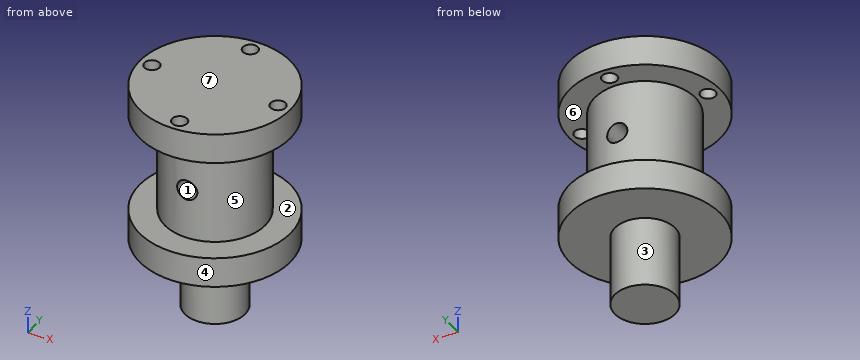
from build123d import *

# Parameters (mm, degrees)
BOSS_EXTRUDE1_DEPTH      = 5
BOSS_EXTRUDE1_DEPTH_BACK = 5
SKETCH1_R                = 5
SKETCH3_R                = 7.5
BOSS_EXTRUDE2_DEPTH      = 3
SKETCH4_R                = 1
CUT_EXTRUDE1_DEPTH       = 17.628289148
SKETCH5_R                = 0.75
CUT_EXTRUDE2_DEPTH       = 17.777961736
CIRPATTERN1_COUNT        = 4
SKETCH6_R                = 3
BOSS_EXTRUDE3_DEPTH      = 7


with BuildPart() as part:
    # Sketch1 → Boss-Extrude1 (new, two sides: drawn at the far end of the back side and taken through both)
    with BuildSketch(Plane.XY.offset(-BOSS_EXTRUDE1_DEPTH_BACK)):
        Circle(SKETCH1_R)
    extrude(amount=BOSS_EXTRUDE1_DEPTH + BOSS_EXTRUDE1_DEPTH_BACK)

    # Sketch3 → Boss-Extrude2 (add)
    with BuildSketch(Plane.XY.offset(5)):
        Circle(SKETCH3_R)
    boss_extrude2 = extrude(amount=BOSS_EXTRUDE2_DEPTH)

    # Mirror1: Boss-Extrude2 across plane
    add(boss_extrude2.mirror(Plane.XY))

    # Sketch4 → Cut-Extrude1 (cut, through all)
    with BuildSketch(Plane(origin=(0, 5, 0), x_dir=(1, 0, 0), z_dir=(0, 1, 0))):
        with Locations(Location((0, 0, 0), (0, 0, 270))):
            Circle(SKETCH4_R)
    extrude(amount=-CUT_EXTRUDE1_DEPTH, mode=Mode.SUBTRACT)

    # Sketch5 → Cut-Extrude2 (cut, through all)
    with BuildSketch(Plane(origin=(0, 0, 5), x_dir=(-1, 0, 0), z_dir=(0, 0, -1))):
        with Locations((0, 6.25)):
            Circle(SKETCH5_R)
    cut_extrude2 = extrude(amount=-CUT_EXTRUDE2_DEPTH, mode=Mode.SUBTRACT)

    # CirPattern1: Cut-Extrude2 ×4 about axis
    cirpattern1_axis = Axis((0, 0, 0), (0, 0, 1))
    for i in range(1, CIRPATTERN1_COUNT):
        add(cut_extrude2.rotate(cirpattern1_axis, i * 360 / CIRPATTERN1_COUNT), mode=Mode.SUBTRACT)

    # Sketch6 → Boss-Extrude3 (add)
    with BuildSketch(Plane(origin=(0, 0, -8), x_dir=(-1, 0, 0), z_dir=(0, 0, -1))):
        Circle(SKETCH6_R)
    extrude(amount=BOSS_EXTRUDE3_DEPTH)


solid = part.part
Verification items for the finished model (mm, model axes). Face numbers are marked on the shaded views. A direction names the side the tool comes from. Give positions to 0.01 mm unless a question says otherwise; leave off trailing zeros. Write each loop counter-clockwise with the first axis right and the second up, starting at its lowest first coordinate (ties: lowest second). Pieces come first, ordered by that corner, then holes. Notation, with made-up numbers: M -7,-30 L 1,-30 A7 ccw 1,-25 Z; hole C 44,17 d7. An arc over 180 degrees is marked long. Put each result on its own line as item: value. Start each with the question number.
1. Scan lines: line 1 along Z through (x, y) = (-2.25, 5.25); line 2 along X through (y, z) = (0.5, 7.25); line 3 along Z through (x, y) = (-3, -1.75). Record each from-to range of solid material in increasing order. Write a range as [from, to].
2. Draft check along Z on the marked faces 4, 5, 6 and 7. Enter one of: +Z half, -Z half, draft (parallel to the pull), parting line (faces both ways), or undercut.
3. Section check B-B (y = -2). Record the cut outline in (x, z), and give its area (3 significant figures).
4. Set-up check for the marked faces 1, 2 and 3: record each of +Z, -Z, +X, -X, +Y, -Y from which the full face is reachable in a straight line by a thin tool's end or side.
5. Section check C-C (y = -6.25). Record the cut outline in (x, z), and give its area (3 significant figures).
6. Section check A-A (y = 0). Record the cut outline in (x, z).
7. Go/stop test with flat-tipped pins: pin 1 Ø3 at (x, z) = (2.5, -10.5) entering from +Y; pin 2 Ø1.4 at (x, y) = (6.25, 0) entering from +Z; pin 3 Ø8 at (y, z) = (5, -8) entering from +X. Record where each tip stops, or that it passes through.
Answer list:
1. line 1: [-8, -5], [5, 8]
1. line 2: [-7.48, -6.81], [-5.69, 5.69], [6.81, 7.48]
1. line 3: [-8, 8]
2. face 4: draft
2. face 5: undercut
2. face 6: undercut
2. face 7: +Z half
3. outline: M -7.23,-8 L -2.24,-8 L -2.24,-15 L 2.24,-15 L 2.24,-8 L 7.23,-8 L 7.23,-5 L 4.58,-5 L 4.58,5 L 7.23,5 L 7.23,8 L -7.23,8 L -7.23,5 L -4.58,5 L -4.58,-5 L -7.23,-5 Z; hole C 0,0 d2
3. area: 207 mm2
4. face 1: +Y, -Y
4. face 2: none
4. face 3: -Z
5. outline: M -4.15,-8 L 4.15,-8 L 4.15,-5 L -4.15,-5 Z; M -4.15,5 L -0.75,5 L -0.75,8 L -4.15,8 Z; M 0.75,5 L 4.15,5 L 4.15,8 L 0.75,8 Z
5. area: 45.2 mm2
6. outline: M -7.5,-8 L -3,-8 L -3,-15 L 3,-15 L 3,-8 L 7.5,-8 L 7.5,-5 L 5,-5 L 5,5 L 5.5,5 L 5.5,8 L -5.5,8 L -5.5,5 L -5,5 L -5,-5 L -7.5,-5 Z; M -7.5,5 L -7,5 L -7,8 L -7.5,8 Z; M 7,5 L 7.5,5 L 7.5,8 L 7,8 Z; hole C 0,0 d2
7. pin 1: y = 2.83
7. pin 2: z = -5
7. pin 3: x = 7.43
